```python
from build123d import *

# Parameters (mm, degrees)
CHAMFER1_SIZE      = 0.25
FILLET1_R          = 0.5
CUT_EXTRUDE1_DEPTH = 0.75


with BuildPart() as part:
    # Sketch1 → Revolve1 (revolve)
    with BuildSketch(Plane.XY, mode=Mode.PRIVATE) as revolve1_sk:
        Polygon((0, 0), (-2.2, 0), (-2.2, -1.6), (-1.25, -1.6), (-1.25, -7.7), (0, -7.7), align=None)
    revolve(revolve1_sk.sketch.rotate(Axis((0, -138.087166902, 0), (0, 1, 0)), 180), axis=Axis((0, -138.087166902, 0), (0, 1, 0)))

    # Chamfer1
    chamfer1_edges = [part.edges().sort_by_distance(p)[0] for p in [
        (-1.25, -7.7, 0),
    ]]
    chamfer(chamfer1_edges, length=CHAMFER1_SIZE)

    # Fillet1
    fillet1_edges = [part.edges().sort_by_distance(p)[0] for p in [
        (-2.2, 0, 0),
    ]]
    fillet(fillet1_edges, radius=FILLET1_R)

    # Sketch2 → Cut-Extrude1 (cut)
    with BuildSketch(Plane(origin=(0, 0, 0), x_dir=(1, 0, 0), z_dir=(0, 1, 0))):
        Polygon((-0.375, 0.375), (-0.375, 1.25), (0.375, 1.25), (0.375, 0.375), (1.25, 0.375), (1.25, -0.375), (0.375, -0.375), (0.375, -1.25), (-0.375, -1.25), (-0.375, -0.375), (-1.25, -0.375), (-1.25, 0.375), align=None)
    extrude(amount=-CUT_EXTRUDE1_DEPTH, mode=Mode.SUBTRACT)


solid = part.part
```
CAD build for the part. Positions are in the model's coordinates, mm. A direction names the side the tool comes from. Coordinates: 2 decimals unless noted, no trailing zeros. Order: outer loops, then holes, each group sorted by start corner. A loop starts at its lowest first (then second) coordinate and runs counter-clockwise, first axis right, second up. Notation, with made-up numbers: (31.25, 17) - (74.25, 17) arc R7 cw to (74.25, 21) - close; hole circle Ø10 at (-20.5, -27). An arc over 180 degrees is marked (long way). Answer in a Markdown table with one row per item.
1. Pull direction Z, two halves, no side cores. Call faces 3 (the face through (-0.29, -1.06, -2.18)), 4 (the face through (-1, 0, 1)), 5 (the face through (0, -0.75, 0)): +Z half, -Z half, draft (parallel to the pull), parting line (faces both ways), or undercut.
Answer:
| item | result |
|---|---|
| face 3 | parting line |
| face 4 | draft |
| face 5 | undercut |
2. Flat gauge pins, fed straight in: P1, Ø0.8, axis at x = 0.5, y = 0, coming from the +Z side; P2, Ø2, axis at x = -0.5, z = 0, coming from the +Y side; P3, Ø1, axis at x = 1.5, y = -3, coming from the -Z side; P4, Ø0.6, axis at y = -0.5, z = 0.5, coming from the +X side. Where does each tip first touch, or does it go through?
Answer:
| item | result |
|---|---|
| P1 | z = 2.16 |
| P2 | y = 0 |
| P3 | z = -0.75 |
| P4 | x = 2.19 |
3. Slice it at B-B, the plane z = 0. List the corners of the cut face in (x, y), then the cut area to 3 significant figures.
Answer:
| item | result |
|---|---|
| outline | (-2.2, -1.6) - (-1.25, -1.6) - (-1.25, -7.45) - (-1, -7.7) - (1, -7.7) - (1.25, -7.45) - (1.25, -1.6) - (2.2, -1.6) - (2.2, -0.5) arc R0.5 ccw to (1.7, 0) - (1.25, 0) - (1.25, -0.75) - (-1.25, -0.75) - (-1.25, 0) - (-1.7, 0) arc R0.5 ccw to (-2.2, -0.5) - close |
| area | 20.2 mm² |
4. Drill centre lines: L1, parallel to Z at x = -0.05, y = -6.5; L2, parallel to Y at x = -1.4, z = 0.1; L3, parallel to Z at x = -1.55, y = -0.25. Where is each one in solid material? Low to high. Write a range as from..to.
Answer:
| item | result |
|---|---|
| L1 | -1.25..1.25 |
| L2 | -1.6..0 |
| L3 | -1.47..1.47 |
5. 3-axis set-ups, long thin cutter, end or side, ignore diameter. For faces 1 (the face through (0, -7.7, 0)), 2 (the face through (-1.25, -4.57, -0.05)): which of +Z, -Z, +X, -X, +Y, -Y reach the whole face in a straight line?
Answer:
| item | result |
|---|---|
| face 1 | +Z, -Z, +X, -X, -Y |
| face 2 | -Y |
6. Slice it at C-C, the plane y = -1.5. List the corners of the cut face in (x, z), then the cut area to 3 significant figures.
Answer:
| item | result |
|---|---|
| outline | circle Ø4.4 at (0, 0) |
| area | 15.2 mm² |
7. Slice it at A-A, the plane x = 0. List the corners of the cut face in (y, z).
Answer:
| item | result |
|---|---|
| outline | (-7.7, -1) - (-7.45, -1.25) - (-1.6, -1.25) - (-1.6, -2.2) - (-0.5, -2.2) arc R0.5 ccw to (0, -1.7) - (0, -1.25) - (-0.75, -1.25) - (-0.75, 1.25) - (0, 1.25) - (0, 1.7) arc R0.5 ccw to (-0.5, 2.2) - (-1.6, 2.2) - (-1.6, 1.25) - (-7.45, 1.25) - (-7.7, 1) - close |
